Geometry: final body of the model. Coordinates: model frame, mm. A direction names the side the tool comes from. Coordinates: 2 decimals unless noted, no trailing zeros. Loops run counter-clockwise (first coordinate to the right, second up) from the corner with the lowest first, then second, coordinate; pieces in that order, holes last. Notation, with made-up numbers: (-24.5, -9) - (-2.5, -9) arc R24 ccw to (-2.5, 9) - close; hole circle Ø8 at (41.25, -22). An arc over 180 degrees is marked (long way). Return JSON: item names as keys, results as strings.
from build123d import *

# Parameters (mm, degrees)
F0_W           = 38.1
F0_H           = 401.32
F1_DEPTH       = 0.635
F2_DEPTH       = 13.97
F3_W           = 12.7
F3_H           = 25.4
F4_DEPTH       = 1.524
F5_W           = 12.7
F5_H           = 25.4
F6_DEPTH       = 1.524
F8_DEPTH       = 12.7
F10_DEPTH      = 12.7
F12_DEPTH      = 1.524
F14_DEPTH      = 1.524
F15_W          = 7.62
F15_H          = 44.45
F16_DEPTH      = 25.4
F17_W          = 12.7
F17_H          = 25.4
F18_DEPTH      = 1.524
F20_DEPTH      = 12.7
F22_DEPTH      = 12.7
F24_DEPTH      = 1.524
F26_DEPTH      = 1.524
F27_W          = 7.62
F27_H          = 44.45
F28_DEPTH      = 25.4
F29_R          = 3.175
F30_DEPTH      = 25.4
F31_R          = 1.5875
F32_DEPTH      = 25.4
F32_DEPTH_BACK = 6.35
F33_R          = 1.5875
F34_DEPTH      = 25.4
F34_DEPTH_BACK = 6.35


with BuildPart() as f1:
    # F0 (on Front) → F1 (new body)
    with BuildSketch(Plane.XZ):
        with Locations((-19.05, -200.66)):
            Rectangle(F0_W, F0_H)
    extrude(amount=F1_DEPTH)

    # F2 (add): a face of the model
    f2_faces = [f1.faces().sort_by_distance(p)[0] for p in [
        (0, -0.3175, -200.66),
    ]]
    extrude(f2_faces, amount=F2_DEPTH)

    # F3 (on face) → F4 (join)
    with BuildSketch(Plane.XZ.offset(0.635)):
        with Locations((1.27, -88.9)):
            Rectangle(F3_W, F3_H)
    extrude(amount=F4_DEPTH)

    # F5 (on face) → F6 (join)
    with BuildSketch(Plane.XZ.offset(0.635)):
        with Locations((-25.4, -88.9)):
            Rectangle(F5_W, F5_H)
    extrude(amount=F6_DEPTH)

    # F7 (on face) → F8 (join)
    with BuildSketch(Plane.YZ.offset(7.62)):
        Polygon((-2.159, -77.724), (-2.159, -76.2), (-101.1457036526, -19.05), (-101.1457036526, -20.574), align=None)
    extrude(amount=-F8_DEPTH)

    # F9 (on face) → F10 (join)
    with BuildSketch(Plane(origin=(-31.75, 0, 0), x_dir=(0, -1, 0), z_dir=(-1, 0, 0))):
        Polygon((100.4791929613, -19.434810127), (2.159, -76.2), (2.159, -77.724), (100.4791929613, -20.958810127), align=None)
    extrude(amount=-F10_DEPTH)

    # F11 (on face) → F12 (join)
    with BuildSketch(Plane.YZ.offset(7.62)):
        Polygon((-101.1457036526, -19.05), (-2.159, -76.2), (-2.159, -61.5353031626), (-94.7957036526, -8.0514773719), align=None)
    extrude(amount=-F12_DEPTH)

    # F13 (on face) → F14 (join)
    with BuildSketch(Plane(origin=(-31.75, 0, 0), x_dir=(0, -1, 0), z_dir=(-1, 0, 0))):
        Polygon((2.159, -61.5353031626), (2.159, -76.2), (100.4791929613, -19.434810127), (94.1291929613, -8.4362874989), align=None)
    extrude(amount=-F14_DEPTH)

    # F15 (on face) → F16 (cut)
    with BuildSketch(Plane(origin=(0, -33.5353178842, -58.0848744234), x_dir=(1, 0, 0), z_dir=(0, 0.5, 0.8660254038))):
        with Locations((-22.86, 2.6250738686)):
            Rectangle(F15_W, F15_H)
        with Locations((-1.27, 2.6250738686)):
            Rectangle(F15_W, F15_H)
    extrude(amount=-F16_DEPTH, mode=Mode.SUBTRACT)

    # F17 (on face) → F18 (join)
    with BuildSketch(Plane.XZ.offset(0.635)):
        with Locations((-25.4, -198.12)):
            Rectangle(F17_W, F17_H)
        with Locations((1.27, -198.12)):
            Rectangle(F17_W, F17_H)
    extrude(amount=F18_DEPTH)

    # F19 (on face) → F20 (join)
    with BuildSketch(Plane.YZ.offset(7.62)):
        Polygon((-2.159, -186.944), (-2.159, -185.42), (-73.6493970824, -144.145), (-73.6493970824, -145.669), align=None)
    extrude(amount=-F20_DEPTH)

    # F21 (on face) → F22 (join)
    with BuildSketch(Plane(origin=(-31.75, 0, 0), x_dir=(0, -1, 0), z_dir=(-1, 0, 0))):
        Polygon((73.6493970824, -144.145), (2.159, -185.42), (2.159, -186.944), (73.6493970824, -145.669), align=None)
    extrude(amount=-F22_DEPTH)

    # F23 (on face) → F24 (join)
    with BuildSketch(Plane.YZ.offset(7.62)):
        Polygon((-73.6493970824, -144.145), (-2.159, -185.42), (-2.159, -173.2028803778), (-67.2993970824, -133.1464773719), align=None)
    extrude(amount=-F24_DEPTH)

    # F25 (on face) → F26 (join)
    with BuildSketch(Plane(origin=(-31.75, 0, 0), x_dir=(0, -1, 0), z_dir=(-1, 0, 0))):
        Polygon((2.159, -173.2192523234), (2.159, -185.42), (73.6493970824, -144.145), (67.2993970824, -133.1464773719), align=None)
    extrude(amount=-F26_DEPTH)

    # F27 (on face) → F28 (cut)
    with BuildSketch(Plane(origin=(0, -80.8289651849, -139.9998744234), x_dir=(1, 0, 0), z_dir=(0, 0.5, 0.8660254038))):
        with Locations((-22.86, 63.5352511532)):
            Rectangle(F27_W, F27_H)
        with Locations((-1.27, 63.5352511532)):
            Rectangle(F27_W, F27_H)
    extrude(amount=-F28_DEPTH, mode=Mode.SUBTRACT)

    # F29 (on face) → F30 (cut)
    with BuildSketch(Plane.XZ.offset(0.635)):
        with Locations((-31.75, -394.97)):
            Circle(F29_R)
        with Locations((-31.75, -344.17)):
            Circle(F29_R)
        with Locations((-6.35, -344.17)):
            Circle(F29_R)
        with Locations((-6.35, -394.97)):
            Circle(F29_R)
    extrude(amount=-F30_DEPTH, mode=Mode.SUBTRACT)

    # F31 (on face) → F32 (join, two sides)
    with BuildSketch(Plane(origin=(0, -33.5353178842, -58.0848744234), x_dir=(1, 0, 0), z_dir=(0, 0.5, 0.8660254038))) as f32_sk:
        with Locations((-25.4, -72.2776037297)):
            Circle(F31_R)
        with Locations((1.27, -73.0472239837)):
            Circle(F31_R)
    extrude(amount=F32_DEPTH)
    extrude(f32_sk.sketch, amount=-F32_DEPTH_BACK)

    # F33 (on face) → F34 (join, two sides)
    with BuildSketch(Plane(origin=(0, -80.8289651849, -139.9998744234), x_dir=(1, 0, 0), z_dir=(0, 0.5, 0.8660254038))) as f34_sk:
        with Locations((-25.4, 13.3702511532)):
            Circle(F33_R)
        with Locations((-0.254, 13.3702511532)):
            Circle(F33_R)
    extrude(amount=F34_DEPTH)
    extrude(f34_sk.sketch, amount=-F34_DEPTH_BACK)


solid = f1.part
Item 1: First-contact query: pin 1 Ø22 at (y, z) = (-25, -168.5) entering from -X; pin 2 Ø1.7 at (x, y) = (1.5, -1) entering from +Z; pin 3 Ø10 at (x, y) = (-32, -26.5) entering from -Z. Flat tips, straight axial feed; report the tip coordinate or a pass-through.
Worked out:
{"pin 1": "x = -31.75", "pin 2": "z = 0", "pin 3": "z = -175.77"}
Item 2: Section query C-C, the plane y = -90.5. Count the separate pieces of the cut face and the enclosed holes in it, and give its area (3 significant figures).
Worked out:
{"separate pieces": "4", "enclosed holes": "0", "area": "115 mm^2"}
Item 3: Section query B-B, the plane z = -229. Return loops of the section in (x, y) (3 decimals), and give its area (3 significant figures).
Worked out:
{"outline": "(-38.1, -0.635) - (13.97, -0.635) - (13.97, 0) - (-38.1, 0) - close", "area": "33.1 mm^2"}
Item 4: Ray query, probe 1 along X at (y, z) = (-0.35, -344.17) (3 decimals); probe 2 along Z at (x, y) = (-31.75, -0.5) (3 decimals); probe 3 along Y at (x, z) = (-32, -101) (3 decimals). Return the intervals inside material, ascending. Write a range as from..to.
Worked out:
{"probe 1": "-38.1..-34.925, -28.575..-9.525, -3.175..13.97", "probe 2": "-401.32..-398.145, -391.795..-347.345, -340.995..0", "probe 3": "-0.635..0"}
Item 5: Section query A-A, the plane z = -53. Return loops of the section in (x, y) (3 decimals).
Worked out:
{"outline": "(-38.1, -0.635) - (13.97, -0.635) - (13.97, 0) - (-38.1, 0) - close; (-31.75, -44.982) - (-26.67, -44.982) - (-26.67, -42.343) - (-30.226, -42.343) - (-30.226, -16.943) - (-31.75, -16.943) - close; (2.54, -44.982) - (7.62, -44.982) - (7.62, -16.943) - (6.096, -16.943) - (6.096, -42.343) - (2.54, -42.343) - close"}
Item 6: Reachability of faces 4 (the face through (-6.76, -0.32, -341.02)), 5 (the face through (-5.08, -59, -153)), 6 (the face through (7.62, -51, -41)), 7 (the face through (1, -2.159, -89)), 8 (the face through (-25.958, -46.348, -159.907)) from +Z, -Z, +X, -X, +Y, -Y: full face, straight path, thin tool, end or side. Return the list, or none.
Worked out:
{"face 4": "+Y, -Y", "face 5": "+Z, -Z, -Y", "face 6": "+Z, -Z, +X, -Y", "face 7": "+X, -X, -Y", "face 8": "none"}
Item 7: Mould query, pull axis X, two halves, no side actions, for faces 1 (the face through (1.26, -62.58, -136.08)), 2 (the face through (-30.999, -70.519, -138.723)), 3 (the face through (-31.75, -50, -41)). Classes: +X half, -X half, draft (parallel to the pull), parting line (faces both ways), or undercut.
Worked out:
{"face 1": "undercut", "face 2": "draft", "face 3": "-X half"}
